from build123d import *

# Parameters (mm, degrees)
F1_DEPTH = 25.4


with BuildPart() as f1:
    # F0 (on Front) → F1 (new body)
    with BuildSketch(Plane.XZ):
        with BuildLine():
            Line((30.4357201419, 32.3955157304), (0, 0))
            Line((0, 0), (-34.3912951606, 28.1609892791))
            ThreePointArc((-34.3912951606, 28.1609892791), (-14.951746221, -41.8598588739), (44.45, 0))
            ThreePointArc((44.45, 0), (40.7962636789, 17.6484381701), (30.4357201419, 32.3955157304))
        make_face()
        with BuildLine():
            Line((-34.3912951606, 28.1609892791), (0, 0))
            Line((0, 0), (30.4357201419, 32.3955157304))
            Line((30.4357201419, 32.3955157304), (21.6344162972, 38.8298149812))
            ThreePointArc((21.6344162972, 38.8298149812), (-8.3150736647, 43.6653415188), (-34.3912951606, 28.1609892791))
        make_face()
        with BuildLine():
            Line((-58.9565059896, 48.2759816213), (-34.3912951606, 28.1609892791))
            ThreePointArc((-34.3912951606, 28.1609892791), (-8.3150736647, 43.6653415188), (21.6344162972, 38.8298149812))
            Line((21.6344162972, 38.8298149812), (-33.6167658697, 79.2218576031))
            Line((-33.6167658697, 79.2218576031), (-58.9565059896, 48.2759816213))
        make_face()
        with BuildLine():
            Line((21.6344162972, 38.8298149812), (30.4357201419, 32.3955157304))
            ThreePointArc((30.4357201419, 32.3955157304), (26.2330865304, 35.8835292452), (21.6344162972, 38.8298149812))
        make_face()
    extrude(amount=F1_DEPTH)


solid = f1.part
Design review of the part built by this model. Coordinates are the model's own, in mm. Round coordinates to 2 decimals unless told otherwise and drop trailing zeros. Write each loop counter-clockwise with the first axis right and the second up, starting at its lowest first coordinate (ties: lowest second). Pieces come first, ordered by that corner, then holes. Notation, with made-up numbers: (16.25, 3) - (47.25, 3) arc R16 cw to (47.25, 30) - close; hole circle Ø3 at (88.25, 53). An arc over 180 degrees is marked (long way). Use a Markdown table: item, result. Add a question column.
1. We need section B-B (y = -9.5). State the section outline as (x, z) points.
2. We need section C-C (z = 15). State the section outline as (x, y) points.
3. We need section A-A (x = -43). State the section outline as (y, z) points, then the cut area to 3 significant figures.
4. Mouldability with a two-part tool opening along Z and no side actions: class faces 1 (the face through (-8, -25.4, 5)), 2 (the face through (-46.846, -12.522, 38.359)), 3 (the face through (-46.109, -12.522, 63.966)) as +Z half, -Z half, draft (parallel to the pull), parting line (faces both ways), or undercut.
5. We need section D-D (x = -14). State the section outline as (y, z) points.
6. Wall thickness on probe 1 along X at (y, z) = (-1.25, 1); probe 2 along Z at (x, y) = (39.5, -11.5); probe 3 along X at (y, z) = (-16.5, 20): over which ranges is each line inside the solid? List them lowest first.
7. Clearance check with flat-ended pins moving along their axes: pin 1 (1.5 mm diameter, centred on y = -7.5, z = 59.5, fed in from -X); pin 2 (12 mm diameter, centred on y = -21.5, z = -13, fed in from -X); pin 3 (8 mm diameter, centred on y = -15, z = 46.5, fed in from +X). State where each tip first meets the part, or that it passes through.
Output:
| question | item | result |
|---|---|---|
| 1 | outline | (-58.96, 48.28) - (-34.39, 28.16) arc R44.45 ccw (long way) to (21.63, 38.83) - (-33.62, 79.22) - close |
| 2 | outline | (-41.84, -25.4) - (41.84, -25.4) - (41.84, 0) - (-41.84, 0) - close |
| 3 | outline | (-25.4, -11.26) - (0, -11.26) - (0, 11.26) - (-25.4, 11.26) - close; (-25.4, 35.21) - (0, 35.21) - (0, 67.76) - (-25.4, 67.76) - close |
| 3 | area | 1,400 mm2 |
| 4 | face 1 | draft |
| 4 | face 2 | undercut |
| 4 | face 3 | +Z half |
| 5 | outline | (-25.4, -42.19) - (0, -42.19) - (0, 64.88) - (-25.4, 64.88) - close |
| 6 | probe 1 | x = -44.44 to 44.44 |
| 6 | probe 2 | z = -20.39 to 20.39 |
| 6 | probe 3 | x = -39.7 to 39.7 |
| 7 | pin 1 | stops at x = -50.38 |
| 7 | pin 2 | stops at x = -43.9 |
| 7 | pin 3 | stops at x = 16.61 |
